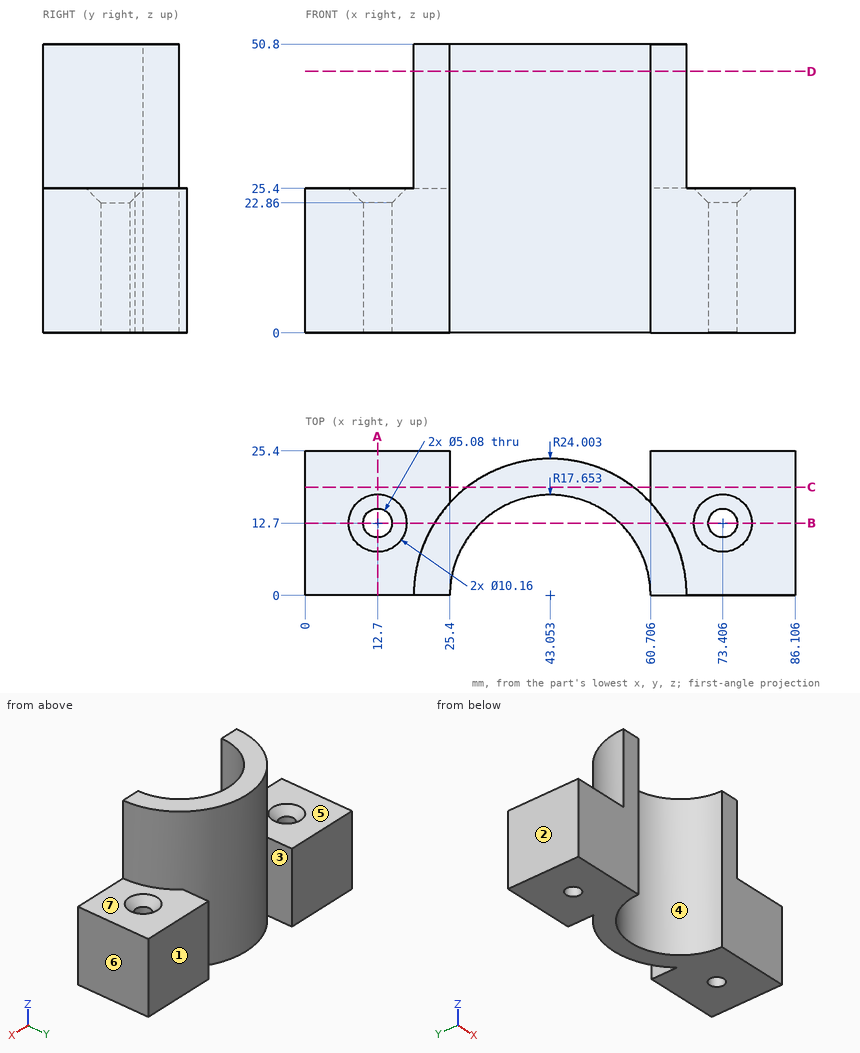
Geometry check sheet. Reference: drawing and pictorial views, mm from the part's lowest x, y, z. A direction names the side the tool comes from. Round coordinates to 2 decimals unless told otherwise and drop trailing zeros. Loops run counter-clockwise (first coordinate to the right, second up) from the corner with the lowest first, then second, coordinate; pieces in that order, holes last.
1. Mould release check, pull along X, two halves, no side actions. Record for the marked faces 1, 2, 3 and 4: released by +X, released by -X, zero draft, split by the parting line, or undercut.
2. Set-up check for the marked faces 5, 6 and 7: record each of +Z, -Z, +X, -X, +Y, -Y from which the full face is reachable in a straight line by a thin tool's end or side.
3. Gauge pin test, flat ends, axial feed: pin 1 Ø3 at (x, z) = (56, 32) entering from -Y; pin 2 Ø3 at (y, z) = (3.5, 32.5) entering from +X; pin 3 Ø7.5 at (x, y) = (79, 12) entering from +Z; pin 4 Ø4 at (x, y) = (12.7, 12.7) entering from -Z. Record the tip position at first contact, or that the pin passes through.
4. Sectioned sample at B-B on y = 12.7. Record the boundary of the cut face in (x, z), and give its area (3 significant figures).
5. Sectioned sample at C-C on y = 19. Record the boundary of the cut face in (x, z), and give its area (3 significant figures).
6. Sectioned sample at A-A on x = 12.7. Record the boundary of the cut face in (y, z).
7. Sectioned sample at D-D on z = 46. Record the boundary of the cut face in (x, y), and give its area (4 significant figures).
8. Scan lines: probe 1 along Y at (x, z) = (12.7, 9); probe 2 along X at (y, z) = (12.7, 17.75); probe 3 along Z at (x, y) = (67.5, 5.5). Record each from-to range of solid material in increasing order.
Recorded:
1. face 1: zero draft
1. face 2: released by -X
1. face 3: undercut
1. face 4: undercut
2. face 5: +Z, -X, +Y
2. face 6: +Z, -Z, +X, +Y, -Y
2. face 7: +Z, +X, +Y
3. pin 1: stops at y = 10.14
3. pin 2: stops at x = 66.97
3. pin 3: stops at z = 25.4
3. pin 4: passes through
4. outline: (0, 0) - (10.16, 0) - (10.16, 22.86) - (7.62, 25.4) - (0, 25.4) - close; (15.24, 0) - (30.79, 0) - (30.79, 50.8) - (22.69, 50.8) - (22.69, 25.4) - (17.78, 25.4) - (15.24, 22.86) - close; (55.31, 0) - (70.87, 0) - (70.87, 22.86) - (68.33, 25.4) - (63.42, 25.4) - (63.42, 50.8) - (55.31, 50.8) - close; (75.95, 0) - (86.11, 0) - (86.11, 25.4) - (78.49, 25.4) - (75.95, 22.86) - close
4. area: 1,710 mm2
5. outline: (0, 0) - (25.4, 0) - (25.4, 25.4) - (0, 25.4) - close; (28.39, 0) - (57.72, 0) - (57.72, 50.8) - (28.39, 50.8) - close; (60.71, 0) - (86.11, 0) - (86.11, 25.4) - (60.71, 25.4) - close
5. area: 2,780 mm2
6. outline: (0, 0) - (10.16, 0) - (10.16, 22.86) - (7.62, 25.4) - (0, 25.4) - close; (15.24, 0) - (25.4, 0) - (25.4, 25.4) - (17.78, 25.4) - (15.24, 22.86) - close
7. outline: (19.05, 0) - (25.4, 0) arc R17.65 cw to (60.71, 0) - (67.06, 0) arc R24 ccw to start
7. area: 415.5 mm2
8. probe 1: y = 0 to 10.16, 15.24 to 25.4
8. probe 2: x = 0 to 10.16, 15.24 to 30.79, 55.31 to 70.87, 75.95 to 86.11
8. probe 3: z = 0 to 25.4
